Autodesk Fusion 360 part; units mm, degrees
sketch "Sketch1" plane through (0, 0, 0) normal (0, 0, 1) x (1, 0, 0)
  line L0 (-0.3848, 44) -> (-43, 44)
  line L1 (-43, 44) -> (-43, -44)
  line L2 (-43, -44) -> (-0.3848, -44)
  line L3 (43, 1.8701) -> (43, -1.8701)
  line L4 (37.435, 11.565) -> (8.8076, 40.1924)
  line L5 (37.435, -11.565) -> (8.8076, -40.1924)
  arc A0 (43, -1.8701) -> (37.435, 11.565) centre (24, -1.8701) ccw
  arc A1 (37.435, -11.565) -> (43, 1.8701) centre (24, 1.8701) ccw
  arc A2 (-0.3848, -44) -> (8.8076, -40.1924) centre (-0.3848, -31) ccw
  arc A3 (8.8076, 40.1924) -> (-0.3848, 44) centre (-0.3848, 31) ccw
  point P0 (43, 6)
  point P1 (5, 44)
  point P2 (43, -6)
  point P3 (5, -44)
  dimension "d2" = 88
  dimension "d7" = 19
  dimension "d8" = 19
  dimension "d9" = 13
  dimension "d10" = 13
extrude "Extrude1" add sketch "Sketch1" along normal blind 10 contours L0 L1 L2 L4 L5 A0 A1 A2 A3 makes body 1
sketch "Sketch3" plane through (0, 0, 10) normal (0, 0, 1) x (-1, 0, 0)
  arc A0 (-37.435, 11.565) -> (-42.9077, 0) centre (-24, -1.8701) ccw
  arc A1 (-42.9077, 0) -> (-37.435, -11.565) centre (-24, 1.8701) ccw
  line L0 (-37.435, -11.565) -> (-8.8076, -40.1924)
  arc A2 (-8.8076, -40.1924) -> (0.3848, -44) centre (0.3848, -31) ccw
  line L1 (0.3848, -44) -> (43, -44)
  line L2 (43, -44) -> (43, 44)
  line L3 (43, 44) -> (0.3848, 44)
  arc A3 (0.3848, 44) -> (-8.8076, 40.1924) centre (0.3848, 31) ccw
  line L4 (-8.8076, 40.1924) -> (-37.435, 11.565)
  line L5 (43, 44) -> (30, 44)
  line L6 (30, -44) -> (43, -44)
  line L7 (27, -19) -> (27, -19)
  line L8 (27, 19) -> (27, 19)
  line L9 (30, -22) -> (30, -44)
  line L10 (30, 44) -> (30, 22)
  arc A4 (30, -22) -> (27, -19) centre (27, -22) ccw
  arc A5 (27, 19) -> (30, 22) centre (27, 22) ccw
  circle A6 centre (43, 0) radius 9.5
  line L11 (43, -44) -> (43, -24.2693)
  line L12 (43, 24.2693) -> (43, 44)
  arc A7 (47.56, -18.4447) -> (47.56, 18.4447) centre (43, 0) ccw
  arc A8 (43, 24.2693) -> (47.56, 18.4447) centre (49, 24.2693) ccw
  arc A9 (47.56, -18.4447) -> (43, -24.2693) centre (49, -24.2693) ccw
  line L13 (27, -5) -> (23, -5)
  line L14 (23, -5) -> (23, 5)
  line L15 (23, 5) -> (27, 5)
  line L16 (27, -19) -> (27, -5)
  line L17 (27, 5) -> (27, 19)
  dimension "d18" = 13
  dimension "d19" = 88
  dimension "d23" = 3
  dimension "d24" = 3
  dimension "d25" = 38
  dimension "d27" = 6
  dimension "d28" = 6
  dimension "d29" = 4
  dimension "d30" = 10
  dimension "d31" = 39
extrude "Extrude2" add sketch "Sketch3" along normal blind 40 separate body contours L1 L2 L3 L5 L6 L9 L10 A4 A5 A6 L11 L12 L13 L14 L15 L16 L17 makes body 2
extrude "Extrude3" add sketch "Sketch3" along normal blind 40 and the other way blind 10 contours L2 A6 A7 A8 A9 bodies 2
sketch "Sketch4" plane through (0, 0, 0) normal (0, 0, 1) x (1, 0, 0)
  line L0 (-43.035, -9.4999) -> (-43.035, 9.4999)
  arc A0 (-43.035, -9.4999) -> (-43.035, 9.4999) centre (-43, 0) ccw
  dimension "d38" = 19
extrude "Extrude4" cut sketch "Sketch4" along normal blind 10 bodies 1
sketch "Sketch5" plane through (0, 0, 0) normal (0, 1, 0) x (1, 0, 0)
  line L0 (-23, -10) -> (31, -10)
  line L1 (31, -10) -> (-23, -50)
  line L2 (-23, -50) -> (-23, -10)
extrude "Extrude5" add sketch "Sketch5" along normal mid plane 10 bodies 1 2
sketch "Sketch6" plane through (0, 0, 10) normal (0, 0, 1) x (-1, 0, 0)
  line L0 (-31, 5) -> (27, 5)
  line L1 (27, 5) -> (27, 19)
  arc A0 (27, 19) -> (30, 22) centre (27, 22) ccw
  line L2 (30, 22) -> (30, 44)
  line L3 (30, 44) -> (0.3848, 44)
  arc A1 (0.3848, 44) -> (-8.8076, 40.1924) centre (0.3848, 31) ccw
  line L4 (-8.8076, 40.1924) -> (-37.435, 11.565)
  arc A2 (-37.435, 11.565) -> (-42.9077, 0) centre (-24, -1.8701) ccw
  arc A3 (-42.9077, 0) -> (-37.435, -11.565) centre (-24, 1.8701) ccw
  line L5 (-37.435, -11.565) -> (-8.8076, -40.1924)
  arc A4 (-8.8076, -40.1924) -> (0.3848, -44) centre (0.3848, -31) ccw
  line L6 (0.3848, -44) -> (30, -44)
  line L7 (30, -44) -> (30, -22)
  arc A5 (30, -22) -> (27, -19) centre (27, -22) ccw
  line L8 (27, -19) -> (27, -5)
  line L9 (27, -5) -> (-31, -5)
  line L10 (-31, -5) -> (-31, 5)
  circle A6 centre (0, 25) radius 5
  circle A7 centre (0, -25) radius 5
  dimension "d43" = 10
  dimension "d44" = 20
  dimension "d45" = 10
extrude "Extrude6" cut sketch "Sketch6" against normal blind 10 contours A6 | A7 bodies 1
equation "d31 = 20 mm + 19 mm"
The model under review builds one solid part; all positions refer to its coordinate system, in mm. A direction names the side the tool comes from. Round coordinates to 2 decimals unless told otherwise and drop trailing zeros. Loops run counter-clockwise (first coordinate to the right, second up) from the corner with the lowest first, then second, coordinate; pieces in that order, holes last. Notation, with made-up numbers: (72.5, 20) - (109.5, 20) arc R18 cw to (109.5, 27) - close; hole circle Ø5 at (16.5, 11). An arc over 180 degrees is marked (long way). Write each question's results on one line, items separated by ' | '. Start each with the question number.
Q1. Insertion check: P1, Ø10, axis at x = -9.5, y = -24, coming from the +Z side; P2, Ø6, axis at y = -30, z = 14.5, coming from the +X side; P3, Ø16, axis at y = 36.5, z = 22.5, coming from the -X side; P4, Ø6, axis at x = 0, y = -25, coming from the -Z side. Each pin has a flat end and moves straight along its axis. Give the tip position at first contact, or say it passes through.
Q2. Take a section at B-B on y = 2.5. Give the boundary of the cut face in (x, z).
Q3. Draft analysis for pull direction X (two halves, no side actions). For faces 5 (the cylindrical face through (-62, 0, 25)), 6 (the cylindrical face through (1.08, 29.88, 5.07)), 7 (the flat face through (23, 26, 5)), 8 (the flat face through (-4, -5, 25)), state which applies: pulls with the +X half, pulls with the -X half, needs draft (parallel to the pull), parting line crosses it, or undercut.
Q4. Take a section at A-A on z = 42. Give the boundary of the cut face in (x, y), plus the area to 3 significant figures.
Q5. Tool access review of faces 1 (the flat face through (-2, 10, 10)), 2 (the flat face through (-27, 12, 30)), 3 (the flat face through (-27, -12, 30)), 4 (the flat face through (-43, 34, 25)): name each direction out of +Z, -Z, +X, -X, +Y, -Y from which nothing blocks a thin tool from reaching the whole face with its end or side.
Q6. Take a section at C-C on y = 37. Give the boundary of the cut face in (x, z), plus the area to 3 significant figures.
Q7. Take a section at D-D on y = 14.5. Give the boundary of the cut face in (x, z).
Q8. Wall thickness on line 1 along Y through (x, z) = (0, 2.5); line 2 along X through (y, z) = (-25, 3.75); line 3 along X through (y, z) = (0, 14.5) (3 decimals): over which ranges is each line inside the solid? List them lowest first. Write a range as [from, to].
Data:
1) P1: stops at z = 10 | P2: stops at x = -30 | P3: stops at x = -43 | P4: passes through
2) outline: (-61.83, 0) - (-52.17, 0) - (-52.17, 50) - (-61.83, 50) - close; (-33.83, 0) - (42.49, 0) - (42.49, 10) - (31, 10) - (-23, 50) - (-33.83, 50) - close
3) face 5: pulls with the -X half | face 6: undercut | face 7: pulls with the +X half | face 8: needs draft
4) outline: (-47.56, -18.44) arc R6 cw to (-43, -24.27) - (-43, -44) - (-30, -44) - (-30, -22) arc R3 cw to (-27, -19) - (-27, -5) - (-12.2, -5) - (-12.2, 5) - (-27, 5) - (-27, 19) arc R3 cw to (-30, 22) - (-30, 44) - (-43, 44) - (-43, 24.27) arc R6 cw to (-47.56, 18.44) arc R19 ccw to start; hole circle Ø19 at (-43, 0) | area: 1,700 mm²
5) face 1: +Z, +X | face 2: +Z, +X, +Y | face 3: +Z, +X, -Y | face 4: +Z, -Z, -X, +Y
6) outline: (-43, 0) - (12, 0) - (12, 10) - (-30, 10) - (-30, 50) - (-43, 50) - close | area: 1,070 mm²
7) outline: (-55.28, 0) - (34.5, 0) - (34.5, 10) - (-27, 10) - (-27, 50) - (-55.28, 50) - close
8) line 1: y = [-43.99, -30], [-20, 20], [30, 43.99] | line 2: x = [-43, -5], [5, 24] | line 3: x = [-62, -52.5], [-33.5, 24.925]
